from build123d import *

# Parameters (mm, degrees)
PAD_DEPTH    = 1
PAD001_DEPTH = 6.5
SKETCH001_W  = 12
SKETCH001_H  = 1
PAD002_DEPTH = 0.5


with BuildPart() as part:
    # Sketch → Pad (new body)
    with BuildSketch(Plane.XY):
        with BuildLine():
            Line((-50.5, 39.25), (50.5, 39.25))
            ThreePointArc((63, 26.75), (59.338835, 35.588835), (50.5, 39.25))
            Line((63, 26.75), (63, -26.75))
            ThreePointArc((50.5, -39.25), (59.338835, -35.588835), (63, -26.75))
            Line((50.5, -39.25), (-50.5, -39.25))
            ThreePointArc((-63, -26.75), (-59.338835, -35.588835), (-50.5, -39.25))
            Line((-63, -26.75), (-63, 26.75))
            ThreePointArc((-50.5, 39.25), (-59.338835, 35.588835), (-63, 26.75))
        make_face()
    extrude(amount=PAD_DEPTH)

    # Sketch → Pad001 (join)
    with BuildSketch(Plane.XY):
        with BuildLine():
            Line((-50.5, 39.25), (50.5, 39.25))
            ThreePointArc((63, 26.75), (59.338835, 35.588835), (50.5, 39.25))
            Line((63, 26.75), (63, -26.75))
            ThreePointArc((50.5, -39.25), (59.338835, -35.588835), (63, -26.75))
            Line((50.5, -39.25), (-50.5, -39.25))
            ThreePointArc((-63, -26.75), (-59.338835, -35.588835), (-50.5, -39.25))
            Line((-63, -26.75), (-63, 26.75))
            ThreePointArc((-50.5, 39.25), (-59.338835, 35.588835), (-63, 26.75))
        make_face()
    extrude(amount=PAD001_DEPTH)

    # Sketch001 (on Face15 of Pad001) → Pad002 (join)
    with BuildSketch(Plane(origin=(0, 39.25, 0), x_dir=(-1, 0, 0), z_dir=(0, 1, 0))):
        with Locations((-20, 0.5)):
            Rectangle(SKETCH001_W, SKETCH001_H)
        with Locations((20, 0.5)):
            Rectangle(SKETCH001_W, SKETCH001_H)
    pad002 = extrude(amount=PAD002_DEPTH)

    # Mirrored: Pad002 across XZ
    add(pad002.mirror(Plane.XZ))


solid = part.part
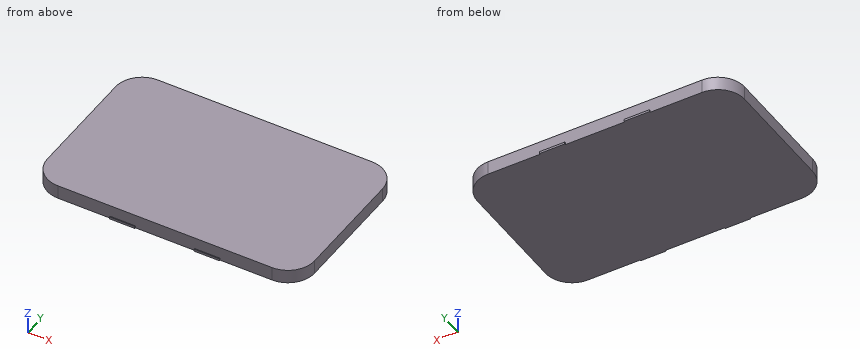
Could you check a few things on this model? Use its own coordinates, in mm. Coordinates: 2 decimals unless noted, no trailing zeros. Order: outer loops, then holes, each group sorted by start corner. A loop starts at its lowest first (then second) coordinate and runs counter-clockwise, first axis right, second up. Notation, with made-up numbers: (-35.75, 82.5) -> (-20.75, 82.5) arc R26 ccw to (-20.75, 100.5) -> close; hole circle Ø3 at (13, 32.5). An arc over 180 degrees is marked (long way). One line per item, written item: value. Start each with the question number.
1) I'm going to push flat-ended pins straight in: pin 1 (0.6 mm diameter, centred on x = 21, y = 39.5, fed in from +Z); pin 2 (1.5 mm diameter, centred on x = 16.5, z = 5, fed in from -Y); pin 3 (2 mm diameter, centred on x = 44, z = 1, fed in from +Y). Where does each tip first touch, or does it pass through?
2) Imagine slicing it at B-B on y = 32.5. List the corners of the cut face in (x, z) for me, plus the area to 3 significant figures.
3) If I drill on L1, parallel to Y at x = -25.5, z = 1.5; L2, parallel to X at y = 35, z = 1; L3, parallel to Y at x = 55, z = 1.75, over which ranges is the centre line in solid material (lowest first)? Write a range as [from, to].
4) Imagine slicing it at A-A on z = 2. List the corners of the cut face in (x, y) for me, plus the area to 3 significant figures.
Answer list:
1. pin 1: stops at z = 6.5
1. pin 2: stops at y = -39.25
1. pin 3: stops at y = 39.25
2. outline: (-61.6, 0) -> (61.6, 0) -> (61.6, 6.5) -> (-61.6, 6.5) -> close
2. area: 801 mm2
3. L1: y = [-39.25, 39.25]
3. L2: x = [-59.89, 59.89]
3. L3: y = [-38.41, 38.41]
4. outline: (-63, -26.75) arc R12.5 ccw to (-50.5, -39.25) -> (50.5, -39.25) arc R12.5 ccw to (63, -26.75) -> (63, 26.75) arc R12.5 ccw to (50.5, 39.25) -> (-50.5, 39.25) arc R12.5 ccw to (-63, 26.75) -> close
4. area: 9,760 mm2
